Geometry: see drawing. Coordinates: mm, zero at the bounding-box minimum. Give positions to 0.01 mm unless a question says otherwise; leave off trailing zeros. Loops run counter-clockwise (first coordinate to the right, second up) from the corner with the lowest first, then second, coordinate; pieces in that order, holes last. Notation, with made-up numbers: (58.5, -12) -> (76.5, -12) arc R11 ccw to (76.5, -2) -> close; hole circle Ø2 at (-34.5, -15.75). An arc over 180 degrees is marked (long way). Return JSON: item names as keys, results as strings. Group by question number.
(1) Cut plane D-D on z = 20.5. Return loops of the section in (x, y).
(2) Ray query, line 1 (X direction, y = 0.7, z = 20); line 2 (Z direction, x = 91.31, y = 0.9); line 3 (X direction, y = 1, z = 59.5). Return the intervals inside material, ascending. Write a range as from..to.
(3) Pin query (flat end, axial travel): pin 1 (12 mm diameter, centred on x = 67, z = 59, fed in from +Y); pin 2 (6.5 mm diameter, centred on x = 10.85, z = 50, fed in from -Y); pin 3 (0.8 mm diameter, centred on x = 35.5, y = 1, fed in from +Z); pin 4 (8 mm diameter, centred on x = 43.5, y = 12.5, fed in from +Z). Return the tip coordinate at first contact, or that it passes through.
(4) Cut plane C-C on y = 14.5. Return loops of the section in (x, z) (1 decimal).
(5) Cut plane B-B on z = 60.5. Return loops of the section in (x, y).
(6) Draft query along X for the marked faces 1, 2 and 3. Return one class per face: released by +X, released by -X, zero draft, split by the parting line, or undercut.
(7) Cut plane A-A on x = 5.58. Return loops of the section in (y, z), then the cut area to 3 significant figures.
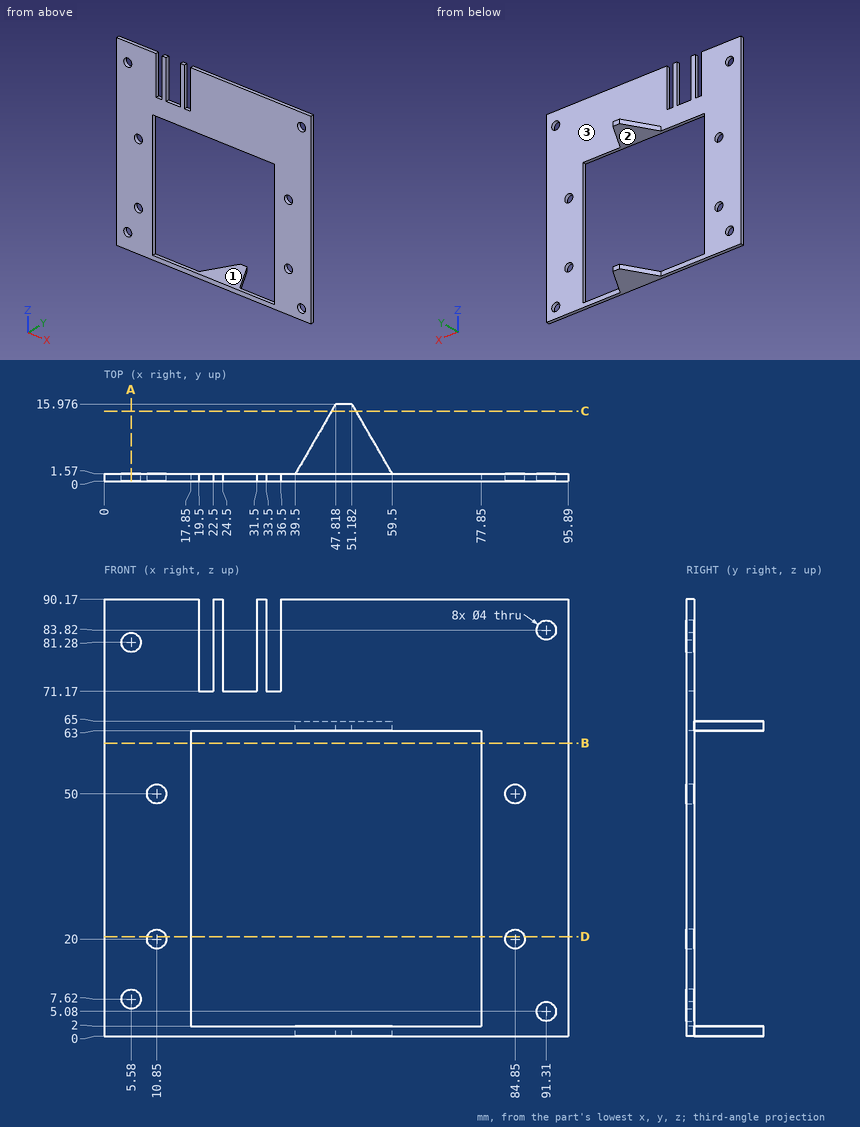
Answers:
{
 "1": {"outline": "(0, 0) -> (8.91, 0) -> (8.91, 1.57) -> (0, 1.57) -> close; (12.79, 0) -> (17.85, 0) -> (17.85, 1.57) -> (12.79, 1.57) -> close; (77.85, 0) -> (82.91, 0) -> (82.91, 1.57) -> (77.85, 1.57) -> close; (86.79, 0) -> (95.89, 0) -> (95.89, 1.57) -> (86.79, 1.57) -> close"},
 "2": {"line 1": "0..8.85, 12.85..17.85, 77.85..82.85, 86.85..95.89", "line 2": "0..3.08, 7.08..81.82, 85.82..90.17", "line 3": "0..17.85, 77.85..95.89"},
 "3": {"pin 1": "y = 1.57", "pin 2": "y = 0", "pin 3": "z = 71.17", "pin 4": "z = 65"},
 "4": {"outline": "(47, 0) -> (52, 0) -> (52, 2) -> (47, 2) -> close; (47, 63) -> (52, 63) -> (52, 65) -> (47, 65) -> close"},
 "5": {"outline": "(0, 0) -> (17.85, 0) -> (17.85, 1.57) -> (0, 1.57) -> close; (77.85, 0) -> (95.89, 0) -> (95.89, 1.57) -> (77.85, 1.57) -> close"},
 "6": {"face 1": "undercut", "face 2": "undercut", "face 3": "zero draft"},
 "7": {"outline": "(0, 0) -> (1.57, 0) -> (1.57, 5.62) -> (0, 5.62) -> close; (0, 9.62) -> (1.57, 9.62) -> (1.57, 79.28) -> (0, 79.28) -> close; (0, 83.28) -> (1.57, 83.28) -> (1.57, 90.17) -> (0, 90.17) -> close", "area": "129 mm²"}
}
